Work out the finished part from the listing and answer in its coordinate system (mm). Face numbers are marked on the shaded views. A direction names the side the tool comes from. Round coordinates to 2 decimals unless told otherwise and drop trailing zeros. Write each loop counter-clockwise with the first axis right and the second up, starting at its lowest first coordinate (ties: lowest second). Pieces come first, ordered by that corner, then holes.
1. Straight lines are drawn through the part: probe 1 along Y at (x, z) = (14.5, 16); probe 2 along Z at (x, y) = (9.5, -75.5); probe 3 along X at (y, z) = (-83.25, 16.75). For each, find the intervals that lie inside material, in ascending order.
2. Find section B-B (x = 24.5). Write down the section's boundary in (y, z), and give its area (3 significant figures).
3. Determine the mould class of the marked faces 4, 5 and 6 for opening direction X: pulls with the +X half, pulls with the -X half, needs draft (parallel to the pull), parting line crosses it, or undercut.
4. Find section C-C (z = 17.5). Write down the section's boundary in (x, y).
5. Flat-ended cylindrical pins translate along their axes: pin 1 Ø2 at (x, y) = (12, -78) entering from +Z; pin 2 Ø1 at (x, y) = (3.5, -81.5) entering from +Z. Find the tip coordinate at first contact, or state that the pin passes through.
6. Find section A-A (y = -77.75). Write down the section's boundary in (x, z).
7. A tool of negligible diameter and unlimited length cuts with its end or side. For the marked faces 1, 2 and 3, from which of +Z, -Z, +X, -X, +Y, -Y can it reach the whole face along a straight path? Write none if from no direction.
8. Find section D-D (z = 22). Write down the section's boundary in (x, y), and give its area (3 significant figures).
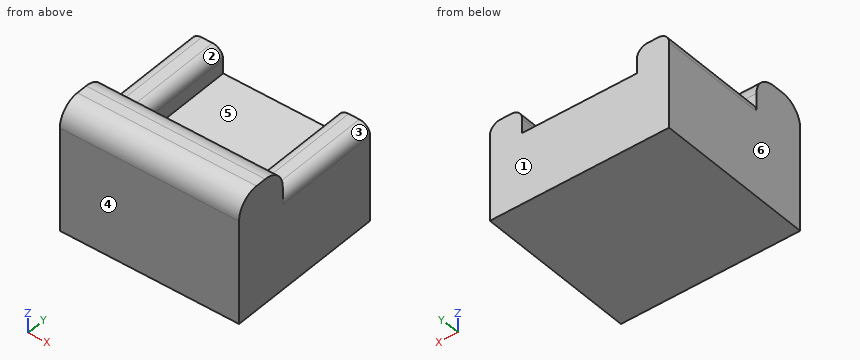
```python
from build123d import *

# Parameters (mm, degrees)
BOX021003023_W     = 33.3333
BOX021003023_H     = 30
BOX021003023_DEPTH = 13.3333
BOX021003025_W     = 6
BOX021003025_H     = 30
BOX021003025_DEPTH = 18
BOX021003026_W     = 6
BOX021003026_H     = 30
BOX021003026_DEPTH = 18
BOX021003020_W     = 33.3333
BOX021003020_H     = 10
BOX021003020_DEPTH = 23.3333
FILLET001_1_R      = 4
FILLET001_2_R      = 2


with BuildPart() as obj1:
    # Box021003023 → Box021003023 (new body)
    with BuildSketch(Plane.XY):
        with Locations((16.66665, 15)):
            Rectangle(BOX021003023_W, BOX021003023_H)
    extrude(amount=BOX021003023_DEPTH)


with BuildPart() as obj2:
    # Box021003025 → Box021003025 (new body)
    with BuildSketch(Plane(origin=(27.3333, 0, 0), x_dir=(1, 0, 0), z_dir=(0, 0, 1))):
        with Locations((3, 15)):
            Rectangle(BOX021003025_W, BOX021003025_H)
    extrude(amount=BOX021003025_DEPTH)


with BuildPart() as obj3:
    # Box021003026 → Box021003026 (new body)
    with BuildSketch(Plane.XY):
        with Locations((3, 15)):
            Rectangle(BOX021003026_W, BOX021003026_H)
    extrude(amount=BOX021003026_DEPTH)


with BuildPart() as obj4:
    # Box021003020 → Box021003020 (new body)
    with BuildSketch(Plane.XY):
        with Locations((16.66665, 5)):
            Rectangle(BOX021003020_W, BOX021003020_H)
    extrude(amount=BOX021003020_DEPTH)

    # Fusion012: union obj1, obj2, obj3
    add(obj1.part)
    add(obj2.part)
    add(obj3.part)

    # Fillet001 1
    fillet001_1_edges = [obj4.edges().sort_by_distance(p)[0] for p in [
        (16.66665, 10, 23.3333),
        (16.66665, 0, 23.3333),
    ]]
    fillet(fillet001_1_edges, radius=FILLET001_1_R)

    # Fillet001 2
    fillet001_2_edges = [obj4.edges().sort_by_distance(p)[0] for p in [
        (0, 20, 18),
        (6, 20, 18),
        (27.3333, 20, 18),
        (33.3333, 20, 18),
    ]]
    fillet(fillet001_2_edges, radius=FILLET001_2_R)


with BuildPart() as obj4_1:
    # Fillet001 placement: moved
    add(obj4.part.moved(Location((0, -100, 0))))


solid = obj4_1.part
```
Worked answers:
1. probe 1: y = -100 to -90
1. probe 2: z = 0 to 13.33
1. probe 3: x = 0.15 to 5.85, 27.48 to 33.19
2. outline: (-100, 0) - (-70, 0) - (-70, 13.33) - (-90, 13.33) - (-90, 19.33) arc R4 ccw to (-94, 23.33) - (-96, 23.33) arc R4 ccw to (-100, 19.33) - close
2. area: 493 mm2
3. face 4: needs draft
3. face 5: undercut
3. face 6: pulls with the -X half
4. outline: (0, -100) - (33.33, -100) - (33.33, -90) - (32.66, -90) - (32.66, -70) - (28.01, -70) - (28.01, -90) - (5.32, -90) - (5.32, -70) - (0.68, -70) - (0.68, -90) - (0, -90) - close
5. pin 1: stops at z = 13.33
5. pin 2: stops at z = 18
6. outline: (0, 0) - (33.33, 0) - (33.33, 16) arc R2 ccw to (31.33, 18) - (29.33, 18) arc R2 ccw to (27.33, 16) - (27.33, 13.33) - (6, 13.33) - (6, 16) arc R2 ccw to (4, 18) - (2, 18) arc R2 ccw to (0, 16) - close
7. face 1: +Z, -Z, +X, -X, +Y
7. face 2: +Z, +Y
7. face 3: +Z, +X, +Y
8. outline: (0, -98.98) - (33.33, -98.98) - (33.33, -91.02) - (0, -91.02) - close
8. area: 265 mm2
